```python
from build123d import *

# Parameters (mm, degrees)
SKETCH_1_R          = 4.5
EXTRUDE_1_DEPTH     = 4.8
SKETCH_2_W          = 11.2
SKETCH_2_H          = 13.8
EXTRUDE_2_DEPTH     = 1.8
SKETCH_4_R          = 2
EXTRUDE_5_DEPTH     = 10
SKETCH_6_W          = 11.2
SKETCH_6_H          = 1
CUT_EXTRUDE_2_DEPTH = 2
FILLET_1_R          = 0.4
SKETCH_3_R          = 3
CUT_EXTRUDE_1_DEPTH = 4
SKETCH_7_R          = 1.5
CUT_EXTRUDE_3_DEPTH = 16.276125163


with BuildPart() as part:
    # Эскиз1 → Бобышка-Вытянуть1 (new body)
    with BuildSketch(Plane.XY):
        Circle(SKETCH_1_R)
    extrude(amount=EXTRUDE_1_DEPTH)

    # Эскиз2 → Бобышка-Вытянуть2 (add)
    with BuildSketch(Plane.XY.offset(4.8)):
        with Locations((0.2, 0.5)):
            Rectangle(SKETCH_2_W, SKETCH_2_H)
    extrude(amount=EXTRUDE_2_DEPTH)

    # Эскиз4 → Бобышка-Вытянуть5 (add)
    with BuildSketch(Plane.XY.offset(6.6)):
        with Locations((-3.35, -1.6)):
            Circle(SKETCH_4_R)
    extrude(amount=EXTRUDE_5_DEPTH)

    # Эскиз6 → Вырез-Вытянуть2 (cut)
    with BuildSketch(Plane.XY.offset(6.6)):
        with Locations((0.2, 6.9)):
            Rectangle(SKETCH_6_W, SKETCH_6_H)
    extrude(amount=-CUT_EXTRUDE_2_DEPTH, mode=Mode.SUBTRACT)

    # Скругление1
    fillet_1_edges = [part.edges().sort_by_distance(p)[0] for p in [
        (-4.5, 0, 0),
    ]]
    fillet(fillet_1_edges, radius=FILLET_1_R)

    # Эскиз3 → Вырез-Вытянуть1 (cut)
    with BuildSketch(Plane(origin=(0, 0, 0), x_dir=(-1, 0, 0), z_dir=(0, 0, -1))):
        Circle(SKETCH_3_R)
    extrude(amount=-CUT_EXTRUDE_1_DEPTH, mode=Mode.SUBTRACT)

    # Эскиз7 → Вырез-Вытянуть3 (cut, through all)
    with BuildSketch(Plane(origin=(0, 0, 4), x_dir=(-1, 0, 0), z_dir=(0, 0, -1))):
        Circle(SKETCH_7_R)
    extrude(amount=-CUT_EXTRUDE_3_DEPTH, mode=Mode.SUBTRACT)


solid = part.part
```
Input: part model. Units: mm. Frame: model coordinates. A direction names the side the tool comes from. Round coordinates to 2 decimals unless told otherwise and drop trailing zeros. Order: outer loops, then holes, each group sorted by start corner. A loop starts at its lowest first (then second) coordinate and runs counter-clockwise, first axis right, second up. Notation, with made-up numbers: (76, -12.75) - (131, -12.75) arc R15 ccw to (131, -6.75) - close; hole circle Ø4 at (9.25, 53). An arc over 180 degrees is marked (long way). Answer in a Markdown table with one row per item.
Item 1: Pin query (flat end, axial travel): pin 1 (1 mm diameter, centred on x = 0, z = 9, fed in from +Y); pin 2 (1.5 mm diameter, centred on x = -3, y = 4, fed in from +Z). Return the tip coordinate at first contact, or that it passes through.
Model answer:
| item | result |
|---|---|
| pin 1 | passes through |
| pin 2 | stops at z = 6.6 |
Item 2: Section query B-B (y = 0). Return the cut outline in (x, z).
Model answer:
| item | result |
|---|---|
| outline | (-5.4, 4.8) - (-4.5, 4.8) - (-4.5, 0.4) arc R0.4 ccw to (-4.1, 0) - (-3, 0) - (-3, 4) - (-1.5, 4) - (-1.5, 6.6) - (-2.15, 6.6) - (-2.15, 16.6) - (-4.55, 16.6) - (-4.55, 6.6) - (-5.4, 6.6) - close; (1.5, 4) - (3, 4) - (3, 0) - (4.1, 0) arc R0.4 ccw to (4.5, 0.4) - (4.5, 4.8) - (5.8, 4.8) - (5.8, 6.6) - (1.5, 6.6) - close |
Item 3: Section query D-D (y = -5). Return the cut outline in (x, z), then the cut area to 3 significant figures.
Model answer:
| item | result |
|---|---|
| outline | (-5.4, 4.8) - (5.8, 4.8) - (5.8, 6.6) - (-5.4, 6.6) - close |
| area | 20.2 mm² |
Item 4: Section query A-A (x = 0). Return the cut outline in (y, z).
Model answer:
| item | result |
|---|---|
| outline | (-6.4, 4.8) - (-4.5, 4.8) - (-4.5, 0.4) arc R0.4 ccw to (-4.1, 0) - (-3, 0) - (-3, 4) - (-1.5, 4) - (-1.5, 6.6) - (-6.4, 6.6) - close; (1.5, 4) - (3, 4) - (3, 0) - (4.1, 0) arc R0.4 ccw to (4.5, 0.4) - (4.5, 4.8) - (6.4, 4.8) - (6.4, 6.6) - (1.5, 6.6) - close |
Item 5: Reachability of faces 5 (the flat face through (4, 3, 4.8)), 6 (the cylindrical face through (-4.937, -2.817, 11.53)), 7 (the flat face through (-5.4, 0, 6)) from +Z, -Z, +X, -X, +Y, -Y: full face, straight path, thin tool, end or side. Return the list, or none.
Model answer:
| item | result |
|---|---|
| face 5 | -Z |
| face 6 | +Z |
| face 7 | +Z, -Z, -X, +Y, -Y |
Item 6: Line query: line 1 (Y direction, x = 0, z = 5.55); line 2 (Y direction, x = 0, z = 1.8); line 3 (Z direction, x = -4.5, y = 1.75). Output: solid intervals per line, ascending.
Model answer:
| item | result |
|---|---|
| line 1 | y = -6.4 to -1.5, 1.5 to 6.4 |
| line 2 | y = -4.5 to -3, 3 to 4.5 |
| line 3 | z = 4.8 to 6.6 |
Item 7: Mould query, pull axis Y, two halves, no side actions, for faces 1 (the cylindrical face through (3, 0, 2)), 2 (the flat face through (0, 6.4, 6)), 3 (the cylindrical face through (1.5, 0.07, 5.28)), 4 (the flat face through (0, -6.4, 6)). Classes: released by +Y, released by -Y, zero draft, split by the parting line, or undercut.
Model answer:
| item | result |
|---|---|
| face 1 | undercut |
| face 2 | released by +Y |
| face 3 | undercut |
| face 4 | released by -Y |
Item 8: Section query C-C (z = 5.75). Return the cut outline in (x, y), then the cut area to 3 significant figures.
Model answer:
| item | result |
|---|---|
| outline | (-5.4, -6.4) - (5.8, -6.4) - (5.8, 6.4) - (-5.4, 6.4) - close; hole circle Ø3 at (0, 0) |
| area | 136 mm² |
